Source: CAD feature listing. Evaluate the final solid. Frame: model axes, mm. A direction names the side the tool comes from. Give positions to 0.01 mm unless a question says otherwise; leave off trailing zeros. Write each loop counter-clockwise with the first axis right and the second up, starting at its lowest first coordinate (ties: lowest second). Pieces come first, ordered by that corner, then holes.
```python
from build123d import *

# Parameters (mm, degrees)
IZIM1_R                     = 7.5
Y_KSEKLIK_EKSTR_ZYON1_DEPTH = 11.75
KES_EKSTR_ZYON1_DEPTH       = 7
RADYUS1_R                   = 1
KES_EKSTR_ZYON2_START       = -2.75
IZIM3_R                     = 3.05
KES_EKSTR_ZYON2_DEPTH       = 2.75


with BuildPart() as part:
    # Çizim1 → Yükseklik-Ekstrüzyon1 (new body)
    with BuildSketch(Plane.XY):
        Circle(IZIM1_R)
    extrude(amount=Y_KSEKLIK_EKSTR_ZYON1_DEPTH)

    # Çizim2 → Kes-Ekstrüzyon1 (cut)
    with BuildSketch(Plane.XY.offset(9.75)):
        with BuildLine():
            Line((-2.655654345, -1.5), (2.655654345, -1.5))
            ThreePointArc((2.655654345, -1.5), (0, 3.05), (-2.655654345, -1.5))
        make_face()
    extrude(amount=-KES_EKSTR_ZYON1_DEPTH, mode=Mode.SUBTRACT)

    # Radyus1
    radyus1_edges = [part.edges().sort_by_distance(p)[0] for p in [
        (-7.5, 0, 0),
        (-7.5, 0, 11.75),
    ]]
    fillet(radyus1_edges, radius=RADYUS1_R)

    # Çizim3 → Kes-Ekstrüzyon2 (cut)
    with BuildSketch(Plane(origin=(0, 0, 0), x_dir=(-1, 0, 0), z_dir=(0, 0, -1)).offset(KES_EKSTR_ZYON2_START)):
        with Locations(Location((0, 0, 0), (0, 0, 209.459174912))):
            Circle(IZIM3_R)
    extrude(amount=KES_EKSTR_ZYON2_DEPTH, mode=Mode.SUBTRACT)


solid = part.part
```
1. Section query A-A (y = 0). Return loops of the section in (x, z), plus the area to 3 significant figures.
2. Access query for faces 1 (the flat face through (0, 0, 11.75)), 2 (the flat face through (0, 0, 9.75)). Directions: +Z, -Z, +X, -X, +Y, -Y. A direction counts if a zero-diameter tool reaches every point of the face in a straight line with its end or side. Return the directions, or none.
3. Section query C-C (z = 4.5). Return loops of the section in (x, y).
4. Pin query (flat end, axial travel): P1, Ø5, axis at x = -4, z = 2, coming from the +Y side; P2, Ø1, axis at x = -5, z = 9.5, coming from the -Y side; P3, Ø5, axis at x = -0.5, y = 0, coming from the -Z side. Return the tip coordinate at first contact, or that it passes through.
5. Line query: probe 1 along Y at (x, z) = (0, 5.5); probe 2 along Z at (x, y) = (-0.5, -2.5); probe 3 along Y at (x, z) = (-2.5, 1.75). Output: solid intervals per line, ascending.
6. Section query B-B (x = 0). Return loops of the section in (y, z).
7. Pull-direction query (X, two-part tool) for faces 3 (the cylindrical face through (-7.493, 0.33, 5.807)), 4 (the flat face through (0, -2, 2.75)), 5 (the flat face through (3, 2, 0)); classes: pulls with the +X half, pulls with the -X half, needs draft (parallel to the pull), parting line crosses it, or undercut.
The answers:
1. outline: (-7.5, 1) arc R1 ccw to (-6.5, 0) - (-3.05, 0) - (-3.05, 9.75) - (3.05, 9.75) - (3.05, 0) - (6.5, 0) arc R1 ccw to (7.5, 1) - (7.5, 10.75) arc R1 ccw to (6.5, 11.75) - (-6.5, 11.75) arc R1 ccw to (-7.5, 10.75) - close
1. area: 116 mm2
2. face 1: +Z, +X, -X, +Y, -Y
2. face 2: -Z
3. outline: circle Ø15 at (0, 0); hole (-2.66, -1.5) - (2.66, -1.5) arc R3.05 ccw (long way) to start
4. P1: stops at y = 7.35
4. P2: stops at y = -6
4. P3: stops at z = 2.75
5. probe 1: y = -7.5 to -1.5, 3.05 to 7.5
5. probe 2: z = 2.75 to 11.75
5. probe 3: y = -7.07 to -1.75, 1.75 to 7.07
6. outline: (-7.5, 1) arc R1 ccw to (-6.5, 0) - (-3.05, 0) - (-3.05, 2.75) - (-1.5, 2.75) - (-1.5, 9.75) - (3.05, 9.75) - (3.05, 0) - (6.5, 0) arc R1 ccw to (7.5, 1) - (7.5, 10.75) arc R1 ccw to (6.5, 11.75) - (-6.5, 11.75) arc R1 ccw to (-7.5, 10.75) - close
7. face 3: parting line crosses it
7. face 4: undercut
7. face 5: needs draft
